Work out the finished part from the listing and answer in its coordinate system (mm). Give positions to 0.01 mm unless a question says otherwise; leave off trailing zeros. Loops run counter-clockwise (first coordinate to the right, second up) from the corner with the lowest first, then second, coordinate; pieces in that order, holes last. Notation, with made-up numbers: (62.25, -26.5) -> (105.25, -26.5) arc R33 ccw to (105.25, 10.5) -> close; hole circle Ø11 at (19.25, 1.25). An arc over 180 degrees is marked (long way). Answer as CSV lines item,"result". Start each with the question number.
1. Find section D-D, the plane x = -9. Give the vertices of the cut face in (y, z).
2. Find the intervals of material crossed by line 1 along Y through (x, z) = (0, 1); line 2 along X through (y, z) = (-1.25, 8); line 3 along Z through (x, y) = (1.5, 3.25), in increasing order.
3. Find section A-A, the plane y = 0. Give the vertices of the cut face in (x, z).
4. Find section C-C, the plane z = 12. Give the vertices of the cut face in (x, y), and give its area (3 significant figures).
5. Determine the mould class of faces 1 (the face through (0, 0, 2.5)), 2 (the face through (-14.985, -0.66, 17.255)), 3 (the face through (-4, 4, 0)) for opening direction Y: +Y half, -Y half, draft (parallel to the pull), parting line (faces both ways), or undercut.
6. Flat-ended cylindrical pins translate along their axes: pin 1 Ø2 at (y, z) = (-11.5, 24) entering from +X; pin 2 Ø3 at (y, z) = (-9, 22.5) entering from +X; pin 3 Ø10 at (x, y) = (-11.5, -12) entering from -Z; pin 4 Ø5 at (x, z) = (-4.5, 34.5) entering from -Y. Find the tip coordinate at first contact, or state that the pin passes through.
Autodesk Fusion 360 part; units mm, degrees
sketch "Esquisse1" plane through (0, 0, 0) normal (0, 0, 1) x (1, 0, 0)
  circle A0 centre (0, 0) radius 15
  dimension "d1" = 30
extrude "Extrusion1" add sketch "Esquisse1" along normal blind 50
fillet "Congé1" radius 15 1 faces at (3.6653, 3.4009, 50)
sketch "Esquisse2" plane through (0, 0, 0) normal (0, 0, 1) x (1, 0, 0)
  circle A0 centre (0, 0) radius 5
  dimension "d6" = 10
extrude "Extrusion2" cut sketch "Esquisse2" along normal blind 2.5
Resolved:
1,outline,"(-12, 0) -> (12, 0) -> (12, 35) arc R12 ccw to (-12, 35) -> close"
2,line 1,"y = -15 to -5, 5 to 15"
2,line 2,"x = -14.95 to 14.95"
2,line 3,"z = 2.5 to 49.57"
3,outline,"(-15, 0) -> (-5, 0) -> (-5, 2.5) -> (5, 2.5) -> (5, 0) -> (15, 0) -> (15, 35) arc R15 ccw to (-15, 35) -> close"
4,outline,"circle Ø30 at (0, 0)"
4,area,"707 mm^2"
5,face 1,"undercut"
5,face 2,"parting line"
5,face 3,"draft"
6,pin 1,"stops at x = 10.71"
6,pin 2,"stops at x = 12.99"
6,pin 3,"stops at z = 0"
6,pin 4,"stops at y = -14.87"
